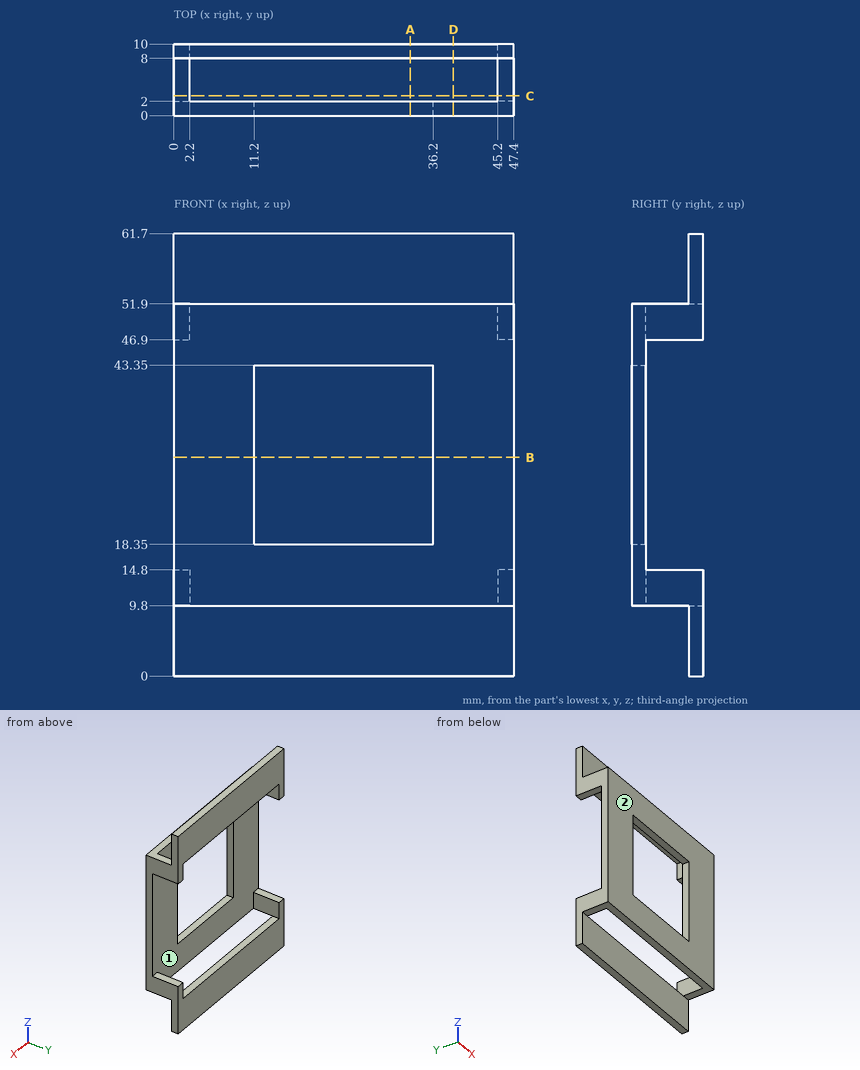
Print and shaded views of the part. All mm, measured from the part's lowest x, y and z. Coordinates: 2 decimals unless noted, no trailing zeros. Order: outer loops, then holes, each group sorted by start corner. A loop starts at its lowest first (then second) coordinate and runs counter-clockwise, first axis right, second up. Notation, with made-up numbers: (74.5, 39.25) -> (79.5, 39.25) arc R38 ccw to (79.5, 78.25) -> close; hole circle Ø2 at (31.5, 62.25). An arc over 180 degrees is marked (long way). Answer as a JSON object with one key per item and string values. Group by question number.
1) Cut at A-A, the plane x = 33. Write the cut outline in (y, z), then the cut area to 3 significant figures.
2) Drill centre lines: L1, parallel to X at y = 1.75, z = 38.5; L2, parallel to X at y = 4.5, z = 12; L3, parallel to Z at x = 8, y = 9. Where is each one in solid material? Low to high.
3) Cut at C-C, the plane y = 2.75. Write the cut outline in (x, z), then the cut area to 3 significant figures.
4) Cut at D-D, the plane x = 39. Write the cut outline in (y, z), then the cut area to 3 significant figures.
5) Flat gauge pins, fed straight in: pin 1 (4 mm diameter, centred on x = 17.5, y = 5.5, fed in from -Z) (3 decimals); pin 2 (3 mm diameter, centred on y = 5, z = 49, fed in from -X); pin 3 (5 mm diameter, centred on x = 40.5, y = 2, fed in from +Z); pin 4 (3 mm diameter, centred on x = 35, z = 18.5, fed in from +Y). Where does each tip first touch, or does it go through?
6) Pull direction X, two halves, no side cores. Call the marked faces 1 and 2: +X half, -X half, draft (parallel to the pull), parting line (faces both ways), or undercut.
7) Cut at B-B, the plane z = 30.5. Write the cut outline in (x, y).
Check values:
{
 "1": {"outline": "(0, 9.8) -> (2, 9.8) -> (2, 18.35) -> (0, 18.35) -> close; (0, 43.35) -> (2, 43.35) -> (2, 51.9) -> (0, 51.9) -> close; (8, 0) -> (10, 0) -> (10, 9.8) -> (8, 9.8) -> close; (8, 51.9) -> (10, 51.9) -> (10, 61.7) -> (8, 61.7) -> close", "area": "73.4 mm²"},
 "2": {"L1": "x = 0 to 11.2, 36.2 to 47.4", "L2": "x = 0 to 2.2, 45.2 to 47.4", "L3": "z = 0 to 9.8, 51.9 to 61.7"},
 "3": {"outline": "(0, 9.8) -> (2.2, 9.8) -> (2.2, 14.8) -> (0, 14.8) -> close; (0, 46.9) -> (2.2, 46.9) -> (2.2, 51.9) -> (0, 51.9) -> close; (45.2, 9.8) -> (47.4, 9.8) -> (47.4, 14.8) -> (45.2, 14.8) -> close; (45.2, 46.9) -> (47.4, 46.9) -> (47.4, 51.9) -> (45.2, 51.9) -> close", "area": "44.0 mm²"},
 "4": {"outline": "(0, 9.8) -> (2, 9.8) -> (2, 51.9) -> (0, 51.9) -> close; (8, 0) -> (10, 0) -> (10, 9.8) -> (8, 9.8) -> close; (8, 51.9) -> (10, 51.9) -> (10, 61.7) -> (8, 61.7) -> close", "area": "123 mm²"},
 "5": {"pin 1": "passes through", "pin 2": "stops at x = 0", "pin 3": "stops at z = 51.9", "pin 4": "stops at y = 2"},
 "6": {"face 1": "undercut", "face 2": "draft"},
 "7": {"outline": "(0, 0) -> (11.2, 0) -> (11.2, 2) -> (0, 2) -> close; (36.2, 0) -> (47.4, 0) -> (47.4, 2) -> (36.2, 2) -> close"}
}
